Verification items for this drawing (mm, ordinates from the low corner). Give positions to 0.01 mm unless a question says otherwise; leave off trailing zeros. Loops run counter-clockwise (first coordinate to the right, second up) from the corner with the lowest first, then second, coordinate; pieces in that order, holes last. Notation, with made-up numbers: M 88.5,14 L 121.5,14 A21 ccw 121.5,36 Z; hole C 17,82.5 d3. An arc over 180 degrees is marked long. Use a Markdown table: item, result.
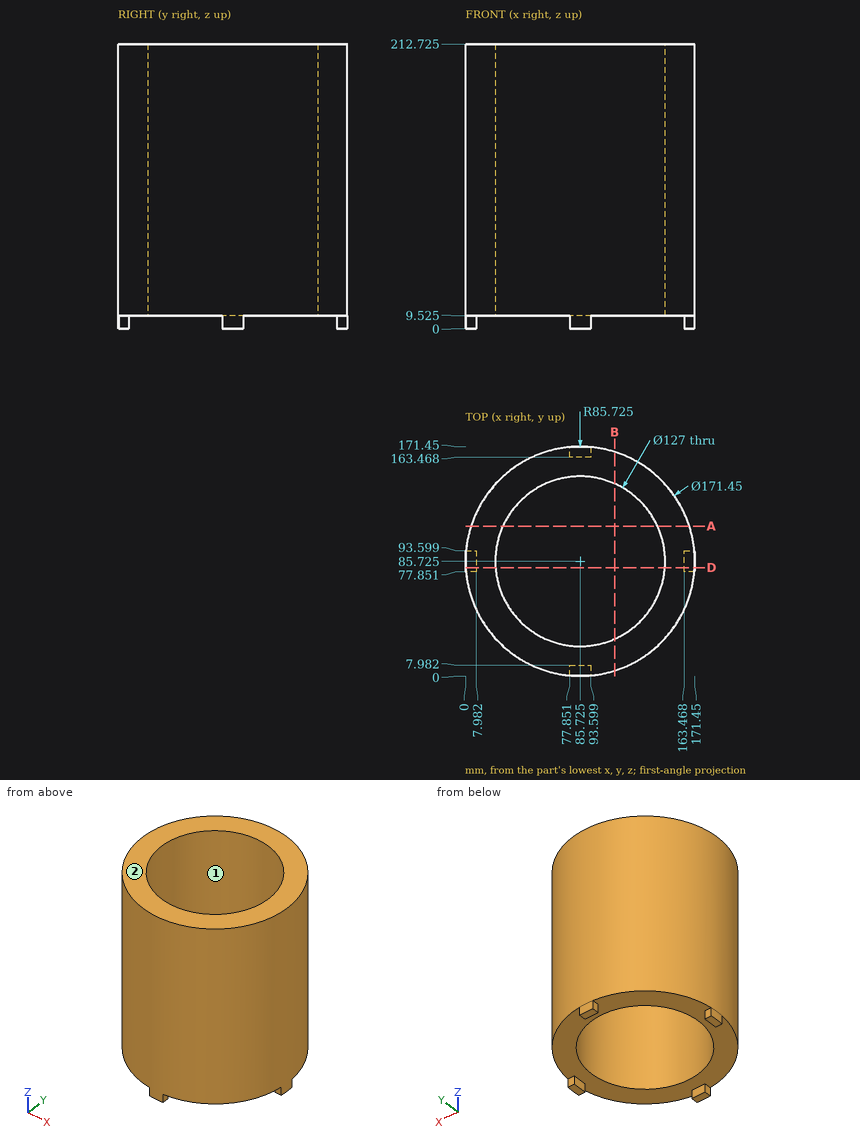
(1) Material ranges on line 1 (Z direction, x = 67, y = 12) (1 decimal); line 2 (X direction, y = 96, z = 75.5); line 3 (X direction, y = 33, z = 48.5) (1 decimal), recorded low to high.
Results below:
| item | result |
|---|---|
| line 1 | 9.5 to 212.7 |
| line 2 | 0.62 to 23.06, 148.39 to 170.83 |
| line 3 | 18.1 to 50.3, 121.1 to 153.3 |
(2) Draft check along Y on the marked faces 1 and 2. Enter one of: +Y half, -Y half, draft (parallel to the pull), parting line (faces both ways), or undercut.
Results below:
| item | result |
|---|---|
| face 1 | undercut |
| face 2 | draft |
(3) Cross-section at D-D on y = 81. Record the cut outline in (x, z) (1 decimal).
Results below:
| item | result |
|---|---|
| outline | M 0.1,0 L 8,0 L 8,9.5 L 22.4,9.5 L 22.4,212.7 L 0.1,212.7 Z; M 149,9.5 L 163.5,9.5 L 163.5,0 L 171.3,0 L 171.3,212.7 L 149,212.7 Z |
(4) Cross-section at B-B on x = 111.5. Record the cut outline in (y, z) (1 decimal).
Results below:
| item | result |
|---|---|
| outline | M 4,9.5 L 27.7,9.5 L 27.7,212.7 L 4,212.7 Z; M 143.8,9.5 L 167.5,9.5 L 167.5,212.7 L 143.8,212.7 Z |
(5) Gauge pin test, flat ends, axial feed: P1, Ø8, axis at x = 34.5, z = 121, coming from the -Y side; P2, Ø3, axis at y = 76.5, z = 185, coming from the -X side; P3, Ø3, axis at y = 89, z = 5.5, coming from the +X side; P4, Ø12, axis at x = 59, y = 143, coming from the +Z side (3 decimals). Record the tip position at first contact, or that the pin passes through.
Results below:
| item | result |
|---|---|
| P1 | y = 14.18 |
| P2 | x = 0.35 |
| P3 | x = 171.43 |
| P4 | z = 212.725 |
(6) Cross-section at A-A on y = 112. Record the cut outline in (x, z) (1 decimal).
Results below:
| item | result |
|---|---|
| outline | M 4.1,9.5 L 27.9,9.5 L 27.9,212.7 L 4.1,212.7 Z; M 143.5,9.5 L 167.3,9.5 L 167.3,212.7 L 143.5,212.7 Z |
